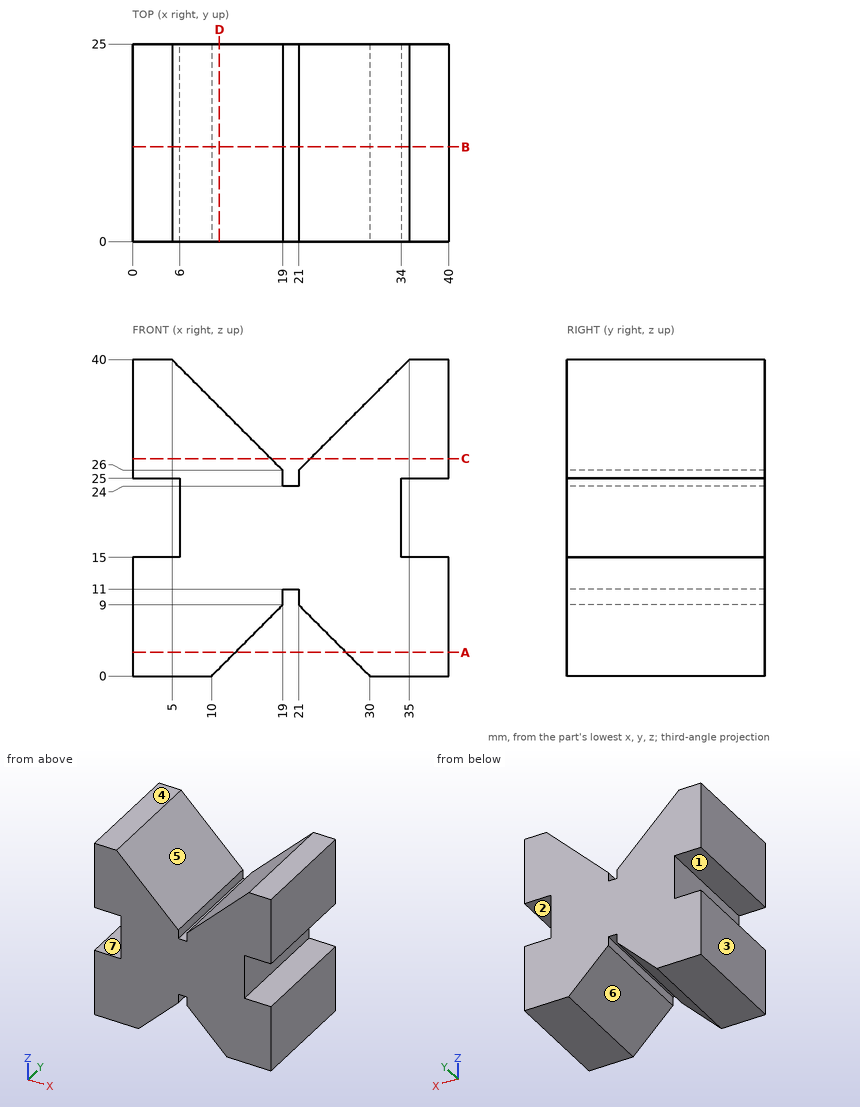
For this review, use the dimensioned drawing (mm, ordinates from the lowest corner) and the shaded views. A direction names the side the tool comes from. Coordinates: 2 decimals unless noted, no trailing zeros. Loops run counter-clockwise (first coordinate to the right, second up) from the corner with the lowest first, then second, coordinate; pieces in that order, holes last. Notation, with made-up numbers: (50, 9) -> (89, 9) arc R21 cw to (89, 32) -> close; hole circle Ø2 at (-30.75, 73.25). An arc over 180 degrees is marked (long way). Use a Markdown table: item, result. Add a question column.
1. Draft analysis for pull direction Z (two halves, no side actions). For the marked faces 1, 2, 3 and 4, state which applies: pulls with the +Z half, pulls with the -Z half, needs draft (parallel to the pull), parting line crosses it, or undercut.
2. Add section C-C on z = 27.5. Write out the cut boundary in (x, y).
3. Add section A-A on z = 3. Write out the cut boundary in (x, y).
4. Add section B-B on y = 12. Write out the cut boundary in (x, z).
5. Add section D-D on x = 11. Write out the cut boundary in (y, z).
6. To check wall thickness, follow line 1 (X direction, y = 18.75, z = 35); line 2 (Z direction, x = 35.5, y = 21); line 3 (X direction, y = 8, z = 27). State the ranges of each line that lie inside material, in increasing order.
7. Machinability: for the marked faces 5, 6 and 7, which of the approach directions +Z, -Z, +X, -X, +Y, -Y give a long, thin tool a straight path to every point of the face, cutting with its end or side? Answer none if there is none.
8. Clearance check with flat-ended pins moving along their axes: pin 1 Ø3 at (x, y) = (5.5, 11) entering from +Z; pin 2 Ø6 at (x, y) = (23.5, 17.5) entering from +Z; pin 3 Ø1.5 at (x, y) = (10, 20) entering from +Z; pin 4 Ø10 at (x, z) = (22, 35) entering from -Y. State where each tip first meets the part, or that it passes through.
Returned:
| question | item | result |
|---|---|---|
| 1 | face 1 | undercut |
| 1 | face 2 | undercut |
| 1 | face 3 | needs draft |
| 1 | face 4 | pulls with the +Z half |
| 2 | outline | (0, 0) -> (17.5, 0) -> (17.5, 25) -> (0, 25) -> close; (22.5, 0) -> (40, 0) -> (40, 25) -> (22.5, 25) -> close |
| 3 | outline | (0, 0) -> (13, 0) -> (13, 25) -> (0, 25) -> close; (27, 0) -> (40, 0) -> (40, 25) -> (27, 25) -> close |
| 4 | outline | (0, 0) -> (10, 0) -> (19, 9) -> (19, 11) -> (21, 11) -> (21, 9) -> (30, 0) -> (40, 0) -> (40, 15) -> (34, 15) -> (34, 25) -> (40, 25) -> (40, 40) -> (35, 40) -> (21, 26) -> (21, 24) -> (19, 24) -> (19, 26) -> (5, 40) -> (0, 40) -> (0, 25) -> (6, 25) -> (6, 15) -> (0, 15) -> close |
| 5 | outline | (0, 1) -> (25, 1) -> (25, 34) -> (0, 34) -> close |
| 6 | line 1 | x = 0 to 10, 30 to 40 |
| 6 | line 2 | z = 0 to 15, 25 to 40 |
| 6 | line 3 | x = 0 to 18, 22 to 40 |
| 7 | face 5 | +Z, +Y, -Y |
| 7 | face 6 | -Z, +Y, -Y |
| 7 | face 7 | -X, +Y, -Y |
| 8 | pin 1 | stops at z = 40 |
| 8 | pin 2 | stops at z = 31.5 |
| 8 | pin 3 | stops at z = 35.75 |
| 8 | pin 4 | passes through |
